Part model, mm, in its own coordinate system. A direction names the side the tool comes from. Coordinates: 2 decimals unless noted, no trailing zeros. Write each loop counter-clockwise with the first axis right and the second up, starting at its lowest first coordinate (ties: lowest second). Pieces come first, ordered by that corner, then holes. Notation, with made-up numbers: (50, -27) -> (88, -27) arc R10 cw to (88, -20) -> close; hole circle Ø6 at (36.5, 71.5). An arc over 180 degrees is marked (long way). Write item = value, one per line. Start each with the question number.
Q1. Pull direction X, two halves, no side cores. Call faces 1 (the flat face through (29, -9.063, 1)), 2 (the flat face through (12.04, -64.04, 0.81)), 3 (the cylindrical face through (-1.5, -0.07, 0.79)), 4 (the cylindrical face through (0, -61, 1)): released by +X, released by -X, zero draft, split by the parting line, or undercut.
Q2. Band-saw the part on C-C, the plane z = 0.3. List the corners of the cut face in (x, y), plus the area to 3 significant figures.
Q3. Pin check, flat tips, straight feed: P1, Ø2.5, axis at x = 0, y = 0, coming from the -Z side; P2, Ø0.8, axis at x = 30.5, z = 0.5, coming from the +Y side; P3, Ø0.5, axis at y = -37, z = 1, coming from the +X side. Stop position of each tip, or through.
Q4. Tool access for faces 5 (the flat face through (28, -61.5, 1)), 6 (the flat face through (29, -50.437, 1)), 7 (the flat face through (28, 2, 1)): list every direction of +Z, -Z, +X, -X, +Y, -Y with a clear straight run to the whole face (end or side of a thin tool).
Q5. Probe line 1 (Y direction, x = 0, z = 1.35); line 2 (Y direction, x = 28, z = 1.15); line 3 (X direction, y = -42.5, z = 0.8). List the from-to ranges inside material, lowest first.
Q6. Band-saw the part on D-D, the plane x = 21. List the corners of the cut face in (y, z), plus the area to 3 significant figures.
Q7. Band-saw the part on B-B, the plane y = 0. List the corners of the cut face in (x, z).
Q8. Band-saw the part on A-A, the plane x = 0. List the corners of the cut face in (y, z).
Autodesk Inventor part; units mm, degrees
ref_plane "YZ Plane" through (0, 0, 0) normal (1, 0, 0) x (0, 1, 0)
ref_plane "XZ Plane" through (0, 0, 0) normal (0, 1, 0) x (-1, 0, 0)
ref_plane "XY Plane" through (0, 0, 0) normal (0, 0, 1) x (1, 0, 0)
sketch "Skizze1" plane through (0, 0, 0) normal (0, 0, 1) x (1, 0, 0)
  arc A0 (3, 7) -> (-3, 1) centre (3, 1) ccw
  line L0 (16.5, 7) -> (3, 7)
  line L1 (16.5, 7) -> (40.4545, 7)
  line L2 (-3, 0) -> (-3, -59.5)
  line L3 (-3, 1) -> (-3, 0)
  arc A1 (-3, -60.5) -> (3, -66.5) centre (3, -60.5) ccw
  line L4 (-3, -59.5) -> (-3, -60.5)
  line L5 (3, -66.5) -> (16.5, -66.5)
  line L6 (16.5, -56.3086) -> (5, -56.3086)
  line L7 (27, -49) -> (27, -62.5)
  line L8 (27, -49) -> (16.5, -49)
  line L9 (16.5, -49) -> (16.5, -56.3086)
  line L10 (16.5, -56.3086) -> (5, -56.3086)
  line L11 (5, -56.3086) -> (5, -37.5)
  line L12 (5, -37.5) -> (3, -37.5)
  line L13 (3, -37.5) -> (3, -22)
  line L14 (3, -22) -> (5, -22)
  line L15 (5, -22) -> (5, -3.0505)
  line L16 (5, -3.0505) -> (16.5, -3.0505)
  line L17 (16.5, -3.0505) -> (16.5, -10.5)
  line L18 (27, -10.5) -> (16.5, -10.5)
  line L19 (27, 3) -> (27, -10.5)
  line L20 (27, 3) -> (16.5, 3)
  line L21 (16.5, 3) -> (16.5, 7)
  line L22 (16.5, 7) -> (3, 7)
  arc A2 (3, 7) -> (-3, 1) centre (3, 1) ccw
  line L23 (-3, 1) -> (-3, 0)
  circle A3 centre (0, 0) radius 3
  line L24 (-3, 0) -> (-3, -59.5)
  circle A4 centre (0, -59.5) radius 3
  line L25 (-3, -59.5) -> (-3, -60.5)
  arc A5 (-3, -60.5) -> (3, -66.5) centre (3, -60.5) ccw
  line L26 (3, -66.5) -> (16.5, -66.5)
  line L27 (16.5, -66.5) -> (16.5, -62.5)
  line L28 (16.5, -62.5) -> (27, -62.5)
  line L29 (-3, 7) -> (16.5, 7)
  line L30 (16.5, -66.5) -> (-3, -66.5)
  line L31 (-3, -66.5) -> (-3, 7)
  line L32 (16.5, 7) -> (41.6272, 7)
  line L33 (41.6272, 7) -> (41.6272, -9.0628)
  line L34 (41.6272, -9.0628) -> (16.5, -9.0628)
  line L35 (16.5, -66.5) -> (41.6272, -66.5)
  line L36 (41.6272, -66.5) -> (41.6272, -50.4372)
  line L37 (41.6272, -50.4372) -> (16.5, -50.4372)
  circle A6 centre (0, 0) radius 1.5
  circle A7 centre (0, -59.5) radius 1.5
  line L38 (16.5, -50.4372) -> (16.5, -9.0628)
  point P0 (0, 0)
  dimension "d5" = 7
  dimension "d6" = 7
extrude "Extrusion1" add sketch "Skizze1" along normal blind 1.6 contours A3 | A4 | L0 L21 L20 L19 L34 L17 L16 L15 L14 L13 L12 L11 L6 L9 L37 L7 L28 L27 L5 A1 L4 L2 L3 A0 | A0 L31 L29 | L1 L32 L33 L34 L19 L20 L21 | A1 L30 L31 | L17 L38 L9 L6 L11 L12 L13 L14 L15 L16 | L27 L28 L7 L37 L36 L35
sketch "Skizze2" plane through (0, 0, 1.6) normal (0, 0, 1) x (1, 0, 0)
  line L0 (-3, -66.5) -> (41.6272, -66.5)
  line L1 (41.6272, -9.0628) -> (41.6272, 7)
  line L2 (41.6272, 7) -> (-3, 7)
  line L3 (41.6272, 2) -> (14.5797, 2)
  line L4 (14.5797, 2) -> (9.5797, 7)
  line L5 (14.5797, 2) -> (21.6508, 2) construction
  dimension "d2" = 135
  dimension "d7" = 5
extrude "Extrusion2" cut sketch "Skizze2" against normal through all
ref_plane "Arbeitsebene1" through (-3, -29.75, 1.6) normal (0, 1, 0) x (1, 0, 0)
mirror "Spiegeln1" about plane through (-3, -29.75, 1.6) normal (0, 1, 0) of "Extrusion2"
properties part number "bottom_sensor"
Ans:
q1.face_1 = zero draft
q1.face_2 = released by +X
q1.face_3 = undercut
q1.face_4 = undercut
q2.outline = (-3, -66.5) -> (9.58, -66.5) -> (14.58, -61.5) -> (41.63, -61.5) -> (41.63, -50.44) -> (16.5, -50.44) -> (16.5, -9.06) -> (41.63, -9.06) -> (41.63, 2) -> (14.58, 2) -> (9.58, 7) -> (-3, 7) -> close; hole circle Ø3 at (0, -59.5); hole circle Ø3 at (0, 0)
q2.area = 1,930 mm2
q3.P1 = through
q3.P2 = 2
q3.P3 = 16.5
q4.face_5 = +Z, -Z, +X, -Y
q4.face_6 = +Z, -Z, +X
q4.face_7 = +Z, -Z, +X, +Y
q5.line_1 = -66.5 to -61, -58 to -1.5, 1.5 to 7
q5.line_2 = -61.5 to -50.44, -9.06 to 2
q5.line_3 = -3 to 16.5
q6.outline = (-61.5, 0) -> (-50.44, 0) -> (-50.44, 1.6) -> (-61.5, 1.6) -> close; (-9.06, 0) -> (2, 0) -> (2, 1.6) -> (-9.06, 1.6) -> close
q6.area = 35.4 mm2
q7.outline = (-3, 0) -> (-1.5, 0) -> (-1.5, 1.6) -> (-3, 1.6) -> close; (1.5, 0) -> (41.63, 0) -> (41.63, 1.6) -> (1.5, 1.6) -> close
q8.outline = (-66.5, 0) -> (-61, 0) -> (-61, 1.6) -> (-66.5, 1.6) -> close; (-58, 0) -> (-1.5, 0) -> (-1.5, 1.6) -> (-58, 1.6) -> close; (1.5, 0) -> (7, 0) -> (7, 1.6) -> (1.5, 1.6) -> close
